Drawing for the job (mm, zero at the part's lowest x, y, z). Round coordinates to 2 decimals unless told otherwise and drop trailing zeros. Order: outer loops, then holes, each group sorted by start corner. A loop starts at its lowest first (then second) coordinate and runs counter-clockwise, first axis right, second up. Notation, with made-up numbers: (-35.5, -21) -> (13.5, -21) arc R34 cw to (13.5, 15) -> close; hole circle Ø7 at (-31.5, 19.25). An arc over 180 degrees is marked (long way). Use CSV: the item, a comma, the result in double quotes.
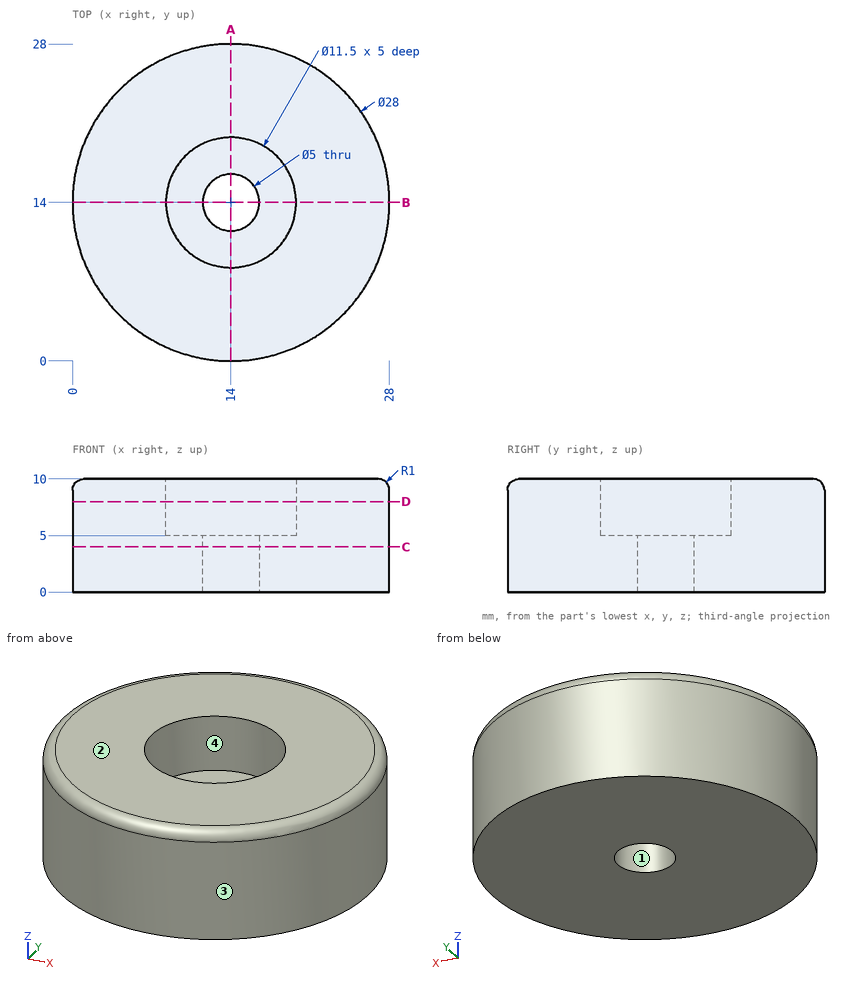
Q1. Cut at D-D (z = 8). Give the cut face in (x, y).
From the geometry:
outline,"circle Ø28 at (14, 14); hole circle Ø11.5 at (14, 14)"
Q2. Pin check, flat tips, straight feed: pin 1 (10.5 mm diameter, centred on x = 14, y = 14, fed in from -Z); pin 2 (6 mm diameter, centred on x = 21.5, z = 2.5, fed in from -Y); pin 3 (6 mm diameter, centred on x = 10.5, z = 3.5, fed in from -Y); pin 4 (1 mm diameter, centred on y = 6.5, z = 8, fed in from -X). Stop position of each tip, or through.
From the geometry:
pin 1,"stops at z = 0"
pin 2,"stops at y = 0.74"
pin 3,"stops at y = 0.01"
pin 4,"stops at x = 1.88"
Q3. Mould opens along Y. For the marked faces 1, 2, 3 and 4 say: +Y half, -Y half, draft (parallel to the pull), parting line (faces both ways), or undercut.
From the geometry:
face 1,"undercut"
face 2,"draft"
face 3,"parting line"
face 4,"undercut"
Q4. Cut at A-A (x = 14). Give the cut face in (y, z), plus the area to 3 significant figures.
From the geometry:
outline,"(0, 0) -> (11.5, 0) -> (11.5, 5) -> (8.25, 5) -> (8.25, 10) -> (1, 10) arc R1 ccw to (0, 9) -> close; (16.5, 0) -> (28, 0) -> (28, 9) arc R1 ccw to (27, 10) -> (19.75, 10) -> (19.75, 5) -> (16.5, 5) -> close"
area,"197 mm²"
Q5. Probe line 1 along Y through (x, z) = (14, 2.6); line 2 along Y through (x, z) = (14, 7.45); line 3 along Z through (x, y) = (16, 18). List the from-to ranges inside material, lowest first.
From the geometry:
line 1,"y = 0 to 11.5, 16.5 to 28"
line 2,"y = 0 to 8.25, 19.75 to 28"
line 3,"z = 0 to 5"
Q6. Cut at C-C (z = 4). Give the cut face in (x, y), plus the area to 3 significant figures.
From the geometry:
outline,"circle Ø28 at (14, 14); hole circle Ø5 at (14, 14)"
area,"596 mm²"
